Read the model definition and answer for the solid it produces. Units are mm, in the model's axes. A direction names the side the tool comes from. Give positions to 0.01 mm unless a question says otherwise; leave off trailing zeros. Order: outer loops, then holes, each group sorted by start corner. A loop starts at its lowest first (then second) coordinate and runs counter-clockwise, first axis right, second up. Notation, with made-up numbers: (24.25, 77) -> (30.25, 77) arc R20 ccw to (30.25, 96) -> close; hole circle Ø2 at (81.5, 85). An arc over 180 degrees is marked (long way). One line per item, written item: value. Start each with the question number.
from build123d import *

# Parameters (mm, degrees)
F0_W     = 150
F0_H     = 200
F0_W_2   = 130
F0_H_2   = 180
F1_DEPTH = 10
F2_SIZE  = 0.4


with BuildPart() as f1:
    # F0 (on Top) → F1 (new body)
    with BuildSketch(Plane.XY):
        Rectangle(F0_W, F0_H)
        Rectangle(F0_W_2, F0_H_2, mode=Mode.SUBTRACT)
    extrude(amount=F1_DEPTH)

    # F2
    f2_edges = [f1.edges().sort_by_distance(p)[0] for p in [
        (75, 0, 10),
        (0, 100, 10),
        (-75, 0, 10),
        (0, -100, 10),
        (0, 90, 10),
        (65, 0, 10),
        (0, -90, 10),
        (-65, 0, 10),
        (75, 0, 0),
        (0, 100, 0),
        (-75, 0, 0),
        (0, -100, 0),
        (0, 90, 0),
        (65, 0, 0),
        (0, -90, 0),
        (-65, 0, 0),
    ]]
    chamfer(f2_edges, length=F2_SIZE)


solid = f1.part
Item 1: Find section B-B on y = -53. Write down the section's boundary in (x, z), then the cut area to 3 significant figures.
Item 2: Find section A-A on x = -46. Write down the section's boundary in (y, z).
Item 3: A tool of negligible diameter and unlimited length cuts with its end or side. For faces 1 (the flat face through (65, -1, 5)), 2 (the flat face through (75, -1, 5)), from which of +Z, -Z, +X, -X, +Y, -Y can it reach the whole face along a straight path? Write none if from no direction.
Item 4: Find the intervals of material crossed by line 1 (X direction, y = -4, z = 3.5); line 2 (Y direction, x = 44, z = 8.25), in increasing order. Write a range as from..to.
Item 5: For a pull along Y with two mould halves and no side action, classify faces 3 (the flat face through (-1, 100, 5)), 4 (the flat face through (-67, 8, 0)), 5 (the flat face through (-65, -1, 5)) as +Y half, -Y half, draft (parallel to the pull), parting line (faces both ways), or undercut.
Item 6: Find section C-C on z = 7.5. Write down the section's boundary in (x, y), then the cut area to 3 significant figures.
Checks:
1. outline: (-75, 0.4) -> (-74.6, 0) -> (-65.4, 0) -> (-65, 0.4) -> (-65, 9.6) -> (-65.4, 10) -> (-74.6, 10) -> (-75, 9.6) -> close; (65, 0.4) -> (65.4, 0) -> (74.6, 0) -> (75, 0.4) -> (75, 9.6) -> (74.6, 10) -> (65.4, 10) -> (65, 9.6) -> close
1. area: 199 mm2
2. outline: (-100, 0.4) -> (-99.6, 0) -> (-90.4, 0) -> (-90, 0.4) -> (-90, 9.6) -> (-90.4, 10) -> (-99.6, 10) -> (-100, 9.6) -> close; (90, 0.4) -> (90.4, 0) -> (99.6, 0) -> (100, 0.4) -> (100, 9.6) -> (99.6, 10) -> (90.4, 10) -> (90, 9.6) -> close
3. face 1: +Z, -Z
3. face 2: +Z, -Z, +X, +Y, -Y
4. line 1: -75..-65, 65..75
4. line 2: -100..-90, 90..100
5. face 3: +Y half
5. face 4: draft
5. face 5: undercut
6. outline: (-75, -100) -> (75, -100) -> (75, 100) -> (-75, 100) -> close; hole (-65, -90) -> (65, -90) -> (65, 90) -> (-65, 90) -> close
6. area: 6,600 mm2
